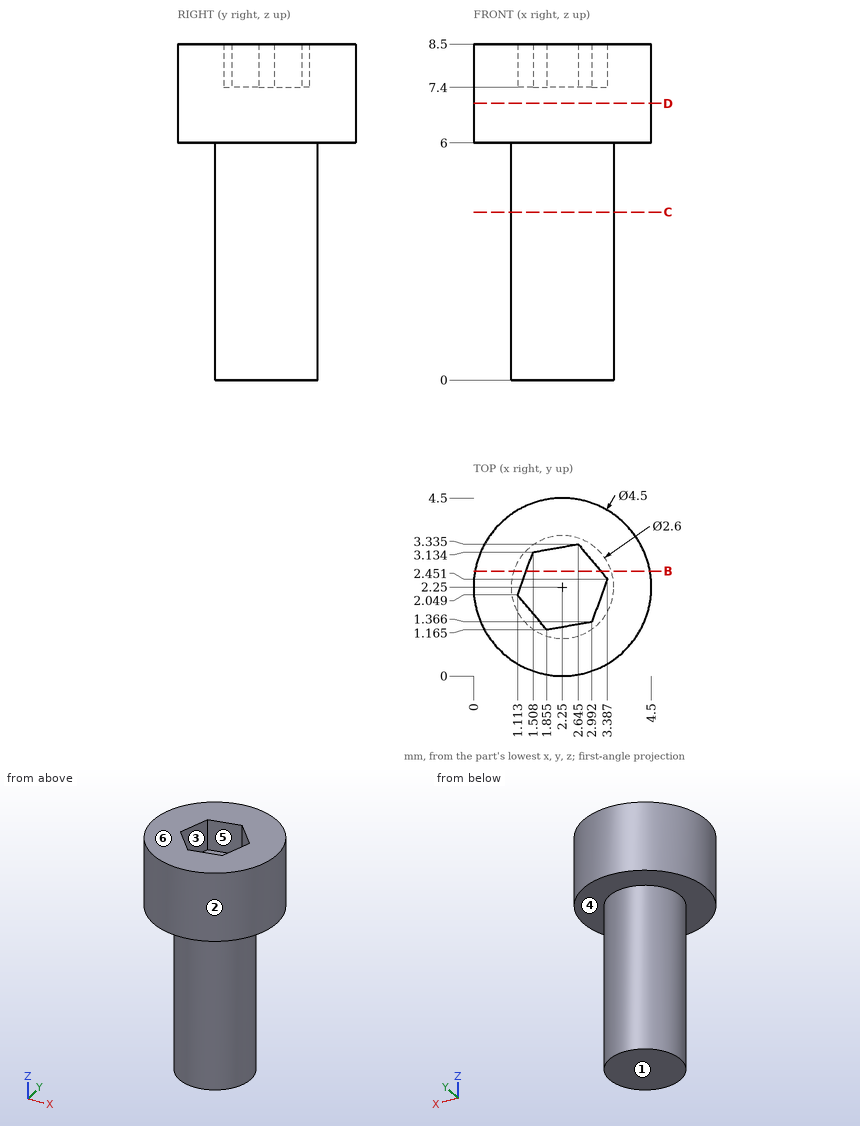
Geometry check sheet. Reference: drawing and pictorial views, mm from the part's lowest x, y, z. A direction names the side the tool comes from. Coordinates: 2 decimals unless noted, no trailing zeros. Order: outer loops, then holes, each group sorted by start corner. A loop starts at its lowest first (then second) coordinate and runs counter-clockwise, first axis right, second up.
Item 1: Section check C-C, the plane z = 4.25. Enter the section's corners in (x, y).
Filled in:
outline: circle Ø2.6 at (2.25, 2.25)
Item 2: Access from +Z, -Z, +X, -X, +Y, -Y to the whole of each face (thin tool, end or side, straight path). Record for the marked faces 4, 5 and 6.
Filled in:
face 4: -Z
face 5: +Z
face 6: +Z, +X, -X, +Y, -Y
Item 3: Section check B-B, the plane y = 2.65. Enter the section's corners in (x, z).
Filled in:
outline: (0.04, 6) - (1.01, 6) - (1.01, 0) - (3.49, 0) - (3.49, 6) - (4.46, 6) - (4.46, 8.5) - (3.22, 8.5) - (3.22, 7.4) - (1.33, 7.4) - (1.33, 8.5) - (0.04, 8.5) - close
Item 4: Material ranges on L1, parallel to Z at x = 2.3, y = 0.5; L2, parallel to Z at x = 2.3, y = 1.7; L3, parallel to Y at x = 1.3, z = 1.75 (1 decimal), recorded low to high.
Filled in:
L1: z = 6 to 8.5
L2: z = 0 to 7.4
L3: y = 1.4 to 3.1
Item 5: Section check D-D, the plane z = 7. Enter the section's corners in (x, y), then the cut area to 3 significant figures.
Filled in:
outline: circle Ø4.5 at (2.25, 2.25)
area: 15.9 mm2
Item 6: Depth check by flat-ended pin: pin 1 (1 mm diameter, centred on x = 2, y = 1.5, fed in from -Z); pin 2 (2 mm diameter, centred on x = 4, z = 4.5, fed in from +Y); pin 3 (1.1 mm diameter, centred on x = 2.5, y = 2.5, fed in from +Z). Enter the tip coordinate at first touch or a pass-through.
Filled in:
pin 1: stops at z = 0
pin 2: stops at y = 3.31
pin 3: stops at z = 7.4
Item 7: Release check for a two-part mould opening along Y. For the marked faces 1, 2 and 3 record: +Y half, -Y half, draft (parallel to the pull), parting line (faces both ways), or undercut.
Filled in:
face 1: draft
face 2: parting line
face 3: undercut
